```python
from build123d import *

# Parameters (mm, degrees)
SKETCH1_R               = 47
BOSS_EXTRUDE1_DEPTH     = 30
SKETCH3_W               = 24
SKETCH3_H               = 15
BOSS_EXTRUDE2_DEPTH     = 30
SKETCH4_W               = 24
SKETCH4_H               = 15
CUT_EXTRUDE1_DEPTH      = 30
CUT_EXTRUDE2_DEPTH      = 81.211785557
CUT_EXTRUDE2_DEPTH_BACK = 30
SKETCH6_R               = 46.5
CUT_EXTRUDE3_DEPTH      = 30
SKETCH9_W               = 4.550783746
SKETCH9_H               = 30
CUT_EXTRUDE4_DEPTH      = 30
SKETCH10_W              = 0.875085896
SKETCH10_H              = 30
CUT_EXTRUDE5_DEPTH      = 30


with BuildPart() as part:
    # Sketch1 → Boss-Extrude1 (new body)
    with BuildSketch(Plane(origin=(0, 0, 0), x_dir=(1, 0, 0), z_dir=(0, 1, 0))):
        with Locations(Location((0, 0, 0), (0, 0, 270))):
            Circle(SKETCH1_R)
    extrude(amount=BOSS_EXTRUDE1_DEPTH)

    # Sketch3 → Boss-Extrude2 (add, symmetric)
    with BuildSketch(Plane(origin=(0, 30, 0), x_dir=(1, 0, 0), z_dir=(0, 1, 0))):
        with Locations((1.837848925, 50.162210695)):
            Rectangle(SKETCH3_W, SKETCH3_H)
    extrude(amount=BOSS_EXTRUDE2_DEPTH, both=True)

    # Sketch4 → Cut-Extrude1 (cut)
    with BuildSketch(Plane(origin=(0, 60, 0), x_dir=(1, 0, 0), z_dir=(0, 1, 0))):
        with Locations((1.837848925, 50.162210695)):
            Rectangle(SKETCH4_W, SKETCH4_H)
    extrude(amount=-CUT_EXTRUDE1_DEPTH, mode=Mode.SUBTRACT)

    # Sketch5 → Cut-Extrude2 (cut, two sides: drawn at the far end of the back side and taken through both)
    with BuildSketch(Plane(origin=(0, 30, 0), x_dir=(1, 0, 0), z_dir=(0, 1, 0)).offset(-CUT_EXTRUDE2_DEPTH_BACK)):
        Polygon((-9.036385525, 57.662210695), (-9.662151075, 57.662210695), (-9.662151075, 45.662210695), (13.337848925, 45.662210695), (13.337848925, 57.662210695), align=None)
    extrude(amount=CUT_EXTRUDE2_DEPTH + CUT_EXTRUDE2_DEPTH_BACK, mode=Mode.SUBTRACT)

    # Sketch6 → Cut-Extrude3 (cut)
    with BuildSketch(Plane(origin=(0, 30, 0), x_dir=(1, 0, 0), z_dir=(0, 1, 0))):
        Circle(SKETCH6_R)
    extrude(amount=-CUT_EXTRUDE3_DEPTH, mode=Mode.SUBTRACT)

    # Sketch9 → Cut-Extrude4 (cut)
    with BuildSketch(Plane(origin=(0, 0, -45.662210695), x_dir=(-1, 0, 0), z_dir=(0, 0, -1))):
        with Locations((-11.062457052, 15)):
            Rectangle(SKETCH9_W, SKETCH9_H)
    extrude(amount=-CUT_EXTRUDE4_DEPTH, mode=Mode.SUBTRACT)

    # Sketch10 → Cut-Extrude5 (cut)
    with BuildSketch(Plane(origin=(0, 0, -45.662210695), x_dir=(-1, 0, 0), z_dir=(0, 0, -1))):
        with Locations((9.224608127, 15)):
            Rectangle(SKETCH10_W, SKETCH10_H)
    extrude(amount=-CUT_EXTRUDE5_DEPTH, mode=Mode.SUBTRACT)


solid = part.part
```
CAD build for the part. Positions are in the model's coordinates, mm. A direction names the side the tool comes from. Coordinates: 2 decimals unless noted, no trailing zeros. Write each loop counter-clockwise with the first axis right and the second up, starting at its lowest first coordinate (ties: lowest second). Pieces come first, ordered by that corner, then holes. Notation, with made-up numbers: (89.25, -26.5) -> (132.25, -26.5) arc R8 ccw to (132.25, -12.5) -> close; hole circle Ø2 at (37, 22). An arc over 180 degrees is marked (long way). Use CSV: the item, a comma, the result in double quotes. Start each with the question number.
Item 1: Tool access for faces 1 (the flat face through (13.338, 15, -51)), 2 (the cylindrical face through (-3.794, 14.79, 46.847)), 3 (the flat face through (13.838, 15, -51)), 4 (the flat face through (-10.162, 15, -52)): list every direction of +Z, -Z, +X, -X, +Y, -Y with a clear straight run to the whole face (end or side of a thin tool).
Item 2: Drop flat-ended pins along their axis: P1, Ø6.5, axis at y = 14, z = -52, coming from the -X side; P2, Ø3.5, axis at y = 21.5, z = -54, coming from the +X side; P3, Ø12, axis at x = -7, y = 11.5, coming from the +Z side. Give the stop position or say it passes through.
Item 3: Band-saw the part on D-D, the plane x = 0. Write the cut outline in (y, z), plus the area to 3 significant figures.
Item 4: Band-saw the part on C-C, the plane y = 12.5. Write the cut outline in (x, z).
Item 5: Band-saw the part on A-A, the plane z = 0. Write the cut outline in (x, y).
Item 6: Band-saw the part on B-B, the plane x = -38. Write the cut outline in (y, z).
Item 7: Wall check: probe 1 along Z at (x, y) = (0, 18.75); probe 2 along X at (y, z) = (21.25, 22); probe 3 along X at (y, z) = (6.75, 2.5). Give the ranges that are in metal, low to high.
Response values:
1,face 1,"-Z, +Y, -Y"
1,face 2,"+Y, -Y"
1,face 3,"-Z, +X, +Y, -Y"
1,face 4,"-Z, -X, +Y, -Y"
2,P1,"stops at x = -10.16"
2,P2,"stops at x = 13.84"
2,P3,"stops at z = 46.99"
3,outline,"(0, 46.5) -> (30, 46.5) -> (30, 47) -> (0, 47) -> close"
3,area,"15.0 mm2"
4,outline,"(-10.16, -57.66) -> (-9.66, -57.66) -> (-9.66, -45.49) arc R46.5 cw (long way) to (13.34, -44.55) -> (13.34, -57.66) -> (13.84, -57.66) -> (13.84, -44.92) arc R47 ccw (long way) to (-10.16, -45.89) -> close"
5,outline,"(-47, 0) -> (-46.5, 0) -> (-46.5, 30) -> (-47, 30) -> close; (46.5, 0) -> (47, 0) -> (47, 30) -> (46.5, 30) -> close"
6,outline,"(0, -27.66) -> (30, -27.66) -> (30, -26.8) -> (0, -26.8) -> close; (0, 26.8) -> (30, 26.8) -> (30, 27.66) -> (0, 27.66) -> close"
7,probe 1,"z = 46.5 to 47"
7,probe 2,"x = -41.53 to -40.97, 40.97 to 41.53"
7,probe 3,"x = -46.93 to -46.43, 46.43 to 46.93"
